Geometry check sheet. Reference: the model listing, model coordinates, mm. Round coordinates to 2 decimals unless told otherwise and drop trailing zeros. Loops run counter-clockwise (first coordinate to the right, second up) from the corner with the lowest first, then second, coordinate; pieces in that order, holes last. Notation, with made-up numbers: (63, 85.25) - (115, 85.25) arc R11 cw to (115, 103.25) - close; hole circle Ø1 at (-26, 76.5). An arc over 180 degrees is marked (long way). Answer in a Markdown table with one row per item. Add a question column.
```python
from build123d import *

# Parameters (mm, degrees)
BOSS_EXTRUDE1_DEPTH   = 5.08
SKETCH2_R             = 22.225
SKETCH2_R_2           = 5.55625
CUT_EXTRUDE1_DEPTH    = 6.08
F_6_CLEARANCE_HOLE1_D = 3.7973


with BuildPart() as part:
    # Sketch1 → Boss-Extrude1 (new body)
    with BuildSketch(Plane.XY):
        Polygon((-84.749075787, 26.84779606), (84.749075787, 26.84779606), (124.522960457, -98.704407881), (39.77388467, -125.55220394), (-39.77388467, -125.55220394), (-124.522960457, -98.704407881), align=None)
    extrude(amount=BOSS_EXTRUDE1_DEPTH)

    # Sketch2 → Cut-Extrude1 (cut, through all)
    with BuildSketch(Plane.XY.offset(5.08)):
        Circle(SKETCH2_R)
        with Locations((-36.5125, 0)):
            Circle(SKETCH2_R_2)
        with Locations((36.5125, 0)):
            Circle(SKETCH2_R_2)
    extrude(amount=-CUT_EXTRUDE1_DEPTH, mode=Mode.SUBTRACT)

    # #6 Clearance Hole1 (through all)
    with Locations(Plane.XY.offset(5.08)):
        with Locations((-73.849633462, 8.68727982), (-103.636097768, -85.338140937), (-55.208054461, -100.679738685), (-34.113357557, -34.091179139), (49.154549048, -102.597438404), (97.582592354, -87.255840656), (28.059852144, -36.008878857), (67.188616869, 8.68727982)):
            Hole(F_6_CLEARANCE_HOLE1_D / 2)


solid = part.part
```
Q1. Cross-section at C-C, the plane y = 0. Enter the section's corners in (x, z) (3 decimals), plus the area to 3 significant figures.
Q2. Cross-section at B-B, the plane z = 1.6. State how many separate pieces and enclosed holes the cut face has, plus the area to 3 significant figures.
Q3. Cross-section at D-D, the plane x = -48. Enter the section's corners in (y, z), plus the area to 3 significant figures.
Q4. Depth check by flat-ended pin: P1, Ø3.5, axis at x = -103.64, y = -85.34, coming from the +Z side; P2, Ø3, axis at y = -7.5, z = 4, coming from the -X side; P3, Ø1, axis at y = -15, z = 2, coming from the +X side. Enter the tip coordinate at first touch or a pass-through.
Q5. Cross-section at A-A, the plane x = 0. Enter the section's corners in (y, z) (3 decimals), plus the area to 3 significant figures.
Q6. Scan lines: line 1 (Y direction, x = -14, z = 0.5); line 2 (X direction, y = 4, z = 0.65); line 3 (X direction, y = -3, z = 0.55). Record each from-to range of solid material in increasing order. Write a range as from..to.
Q7. Release check for a two-part mould opening along X. For faces 1 (the cylindrical face through (21.199, 6.676, 2.576)), 2 (the flat face through (-81.6, -112.3, 2.5)), 3 (the flat face through (2, -48, 0)) record: +X half, -X half, draft (parallel to the pull), parting line (faces both ways), or undercut.
Check sheet entries:
| question | item | result |
|---|---|---|
| 1 | outline | (-93.254, 0) - (-42.069, 0) - (-42.069, 5.08) - (-93.254, 5.08) - close; (-30.956, 0) - (-22.225, 0) - (-22.225, 5.08) - (-30.956, 5.08) - close; (22.225, 0) - (30.956, 0) - (30.956, 5.08) - (22.225, 5.08) - close; (42.069, 0) - (93.254, 0) - (93.254, 5.08) - (42.069, 5.08) - close |
| 1 | area | 609 mm² |
| 2 | separate pieces | 1 |
| 2 | enclosed holes | 11 |
| 2 | area | 28,800 mm² |
| 3 | outline | (-122.95, 0) - (26.85, 0) - (26.85, 5.08) - (-122.95, 5.08) - close |
| 3 | area | 761 mm² |
| 4 | P1 | through |
| 4 | P2 | x = -96.11 |
| 4 | P3 | x = 98.16 |
| 5 | outline | (-125.552, 0) - (-22.225, 0) - (-22.225, 5.08) - (-125.552, 5.08) - close; (22.225, 0) - (26.848, 0) - (26.848, 5.08) - (22.225, 5.08) - close |
| 5 | area | 548 mm² |
| 6 | line 1 | -125.55..-17.26, 17.26..26.85 |
| 6 | line 2 | -91.99..-40.37, -32.66..-21.86, 21.86..32.66, 40.37..91.99 |
| 6 | line 3 | -94.2..-41.19, -31.84..-22.02, 22.02..31.84, 41.19..94.2 |
| 7 | face 1 | undercut |
| 7 | face 2 | -X half |
| 7 | face 3 | draft |
